Design review of the part built by this model. Coordinates are the model's own, in mm. Give positions to 0.01 mm unless a question says otherwise; leave off trailing zeros. Write each loop counter-clockwise with the first axis right and the second up, starting at its lowest first coordinate (ties: lowest second). Pieces come first, ordered by that corner, then holes.
Autodesk Inventor part; units mm, degrees
ref_plane "YZ Plane" through (0, 0, 0) normal (1, 0, 0) x (0, 1, 0)
ref_plane "XZ Plane" through (0, 0, 0) normal (0, 1, 0) x (-1, 0, 0)
ref_plane "XY Plane" through (0, 0, 0) normal (0, 0, 1) x (1, 0, 0)
sketch "Sketch1" plane through (0, 0, 0) normal (0, 1, 0) x (-1, 0, 0)
  line L0 (-87, 87) -> (87, 87) construction
  line L1 (87, 87) -> (87, -87) construction
  line L2 (87, -87) -> (-87, -87) construction
  line L3 (-87, -87) -> (-87, 87) construction
  line L4 (-87, 87) -> (87, -87) construction
  line L5 (87, 87) -> (-87, -87) construction
  line L6 (-90, 90) -> (90, 90)
  line L7 (90, 90) -> (90, -90)
  line L8 (90, -90) -> (-90, -90)
  line L9 (-90, -90) -> (-90, 90)
  line L10 (-90, 90) -> (90, -90) construction
  line L11 (90, 90) -> (-90, -90) construction
  point P0 (0, 0)
  dimension "d0" = 174
  dimension "d1" = 174
  dimension "d2" = 3
extrude "Extrusion1" add sketch "Sketch1" along normal blind 3
sketch "Sketch2" plane through (0, 3, 0) normal (0, 1, 0) x (1, 0, 0)
  circle A0 centre (0, 0) radius 25
  dimension "d5" = 50
extrude "Extrusion2" cut sketch "Sketch2" against normal through all
properties part number "Tapa"
(1) Consider section A-A, the plane z = 0. Give the boundary of the cut face in (x, y), then the cut area to 3 significant figures.
Resolved:
outline: (-90, 0) - (-25, 0) - (-25, 3) - (-90, 3) - close; (25, 0) - (90, 0) - (90, 3) - (25, 3) - close
area: 390 mm2
(2) Consider section C-C, the plane y = 2.2. Give the boundary of the cut face in (x, z).
Resolved:
outline: (-90, -90) - (90, -90) - (90, 90) - (-90, 90) - close; hole circle Ø50 at (0, 0)
(3) Clearance check with a flat-ended pin moving along its axis: P1, Ø10, axis at x = -19, z = 14, coming from the +Y side. State where the tip first meets the part, or that it passes through.
Resolved:
P1: stops at y = 3
(4) Consider section B-B, the plane x = 0. Give the boundary of the cut face in (y, z).
Resolved:
outline: (0, -90) - (3, -90) - (3, -25) - (0, -25) - close; (0, 25) - (3, 25) - (3, 90) - (0, 90) - close
(5) Mouldability with a two-part tool opening along Z and no side actions: class faces 1 (the face through (23.846, 1.521, -7.509)), 2 (the face through (-19, 0, 21)) as pulls with the +Z half, pulls with the -Z half, needs draft (parallel to the pull), parting line crosses it, or undercut.
Resolved:
face 1: undercut
face 2: needs draft
(6) To check wall thickness, follow L1, parallel to X at y = 0.8, z = 0; L2, parallel to X at y = 0.55, z = -13.5. State the ranges of each line that lie inside material, in increasing order.
Resolved:
L1: x = -90 to -25, 25 to 90
L2: x = -90 to -21.04, 21.04 to 90
